Can you work these out from the model? Positions are in its coordinate system, mm. Face numbers are marked on the shaded views. A direction names the side the tool comes from. Give positions to 0.01 mm unless a question says otherwise; leave off trailing zeros. Write each loop counter-clockwise with the first axis right and the second up, starting at its lowest first coordinate (ties: lowest second). Pieces come first, ordered by that corner, then holes. Notation, with made-up numbers: M 2,-35.75 L 41,-35.75 A8 cw 41,-30.75 Z; hole C 69.5,5 d3. An arc over 180 degrees is marked long. Write each question's results on one line, items separated by ' | '.
Autodesk Fusion 360 part; units mm, degrees
sketch "Sketch1" plane through (0, 0, 0) normal (0, 1, 0) x (1, 0, 0)
  line L0 (16, 9.2376) -> (0, 18.4752)
  line L1 (0, 18.4752) -> (-16, 9.2376)
  line L2 (-16, 9.2376) -> (-16, -9.2376)
  line L3 (-16, -9.2376) -> (0, -18.4752)
  line L4 (0, -18.4752) -> (16, -9.2376)
  line L5 (16, -9.2376) -> (16, 9.2376)
  line L6 (13, 7.5056) -> (0, 15.0111)
  line L7 (0, 15.0111) -> (-13, 7.5056)
  line L8 (-13, 7.5056) -> (-13, -7.5056)
  line L9 (-13, -7.5056) -> (0, -15.0111)
  line L10 (0, -15.0111) -> (13, -7.5056)
  line L11 (13, -7.5056) -> (13, 7.5056)
  dimension "d1" = 16
  dimension "d2" = 3
extrude "Extrude1" add sketch "Sketch1" along normal blind 70 makes body 1
extrude "Extrude2" add sketch "Sketch1" along normal blind 3 contours L6 L7 L8 L9 L10 L11 bodies 1
copy_body "Body->Comp1" bodies 1 removing the originals makes body 2 in component "hexagon-02"
component "hexagon-02" placed x (1, 0, 0) y (0, 1, 0) z (0, 0, 1) at (0, 0, 0)
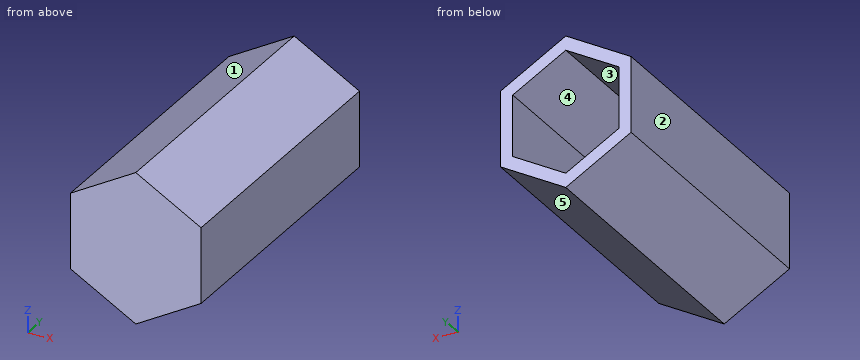
Item 1: I'm going to push flat-ended pins straight in: pin 1 (10 mm diameter, centred on x = -6.5, y = 60, fed in from +Z); pin 2 (8 mm diameter, centred on x = 10.5, z = -8, fed in from -Y); pin 3 (6 mm diameter, centred on x = -8.5, y = 55.5, fed in from +Z); pin 4 (1.5 mm diameter, centred on y = 43.5, z = 11, fed in from +X). Where does each tip first touch, or does it pass through?
Geometry says:
pin 1: stops at z = 17.61 | pin 2: stops at y = 0 | pin 3: stops at z = 15.3 | pin 4: stops at x = 14.25
Item 2: If I drill on line 1 (X direction, y = 66, z = 3); line 2 (Y direction, x = 9, z = -8); line 3 (Z direction, x = 9, y = 22), over which ranges is the centre line in solid material (lowest first)? Write a range as from..to.
Geometry says:
line 1: x = -16..-13, 13..16 | line 2: y = 0..3 | line 3: z = -13.28..-9.81, 9.81..13.28
Item 3: I want a section at A-A, the plane y = 66. Please give me the cut outline in (x, z).
Geometry says:
outline: M -16,-9.24 L 0,-18.48 L 16,-9.24 L 16,9.24 L 0,18.48 L -16,9.24 Z; hole M -13,-7.51 L 0,-15.01 L 13,-7.51 L 13,7.51 L 0,15.01 L -13,7.51 Z
Item 4: For the marked faces 4 and 5, which set-ups out of +Z, -Z, +X, -X, +Y, -Y let a thin tool reach every point of the face, with its end or its side?
Geometry says:
face 4: +Y | face 5: -Z, +X, +Y, -Y
Item 5: I want a section at C-C, the plane x = -1.5. Please give me the cut outline in (y, z).
Geometry says:
outline: M 0,-17.61 L 70,-17.61 L 70,-14.15 L 3,-14.15 L 3,14.15 L 70,14.15 L 70,17.61 L 0,17.61 Z
Item 6: I want a section at B-B, the plane z = -2. Please give me the cut outline in (x, y), and give its area (3 significant figures).
Geometry says:
outline: M -16,0 L 16,0 L 16,70 L 13,70 L 13,3 L -13,3 L -13,70 L -16,70 Z | area: 498 mm2
Item 7: Thinking about a two-plate mould opening in Z: for the marked faces 1, 2 and 3, which applies, +Z half, -Z half, draft (parallel to the pull), parting line (faces both ways), or undercut?
Geometry says:
face 1: +Z half | face 2: draft | face 3: undercut
